Work out the finished part from the listing and answer in its coordinate system (mm). A direction names the side the tool comes from. Round coordinates to 2 decimals unless told otherwise and drop trailing zeros. Write each loop counter-clockwise with the first axis right and the second up, starting at its lowest first coordinate (ties: lowest second). Pieces come first, ordered by that corner, then holes. Notation, with made-up numbers: (-21.5, 9) - (11.5, 9) arc R10 cw to (11.5, 13) - close; hole circle Ø10 at (70, 14.5). An arc over 180 degrees is marked (long way). Write item = value, one per line. Start each with the question number.
from build123d import *

# Parameters (mm, degrees)
EXTRUDE1_DEPTH = 8


with BuildPart() as part:
    # Sketch1 → Extrude1 (new body)
    with BuildSketch(Plane(origin=(0, 0, 0), x_dir=(1, 0, 0), z_dir=(0, 1, 0))):
        Polygon((30, 0), (15, 25.980762114), (-15, 25.980762114), (-30, 0), (-15, -25.980762114), (15, -25.980762114), align=None)
    extrude(amount=EXTRUDE1_DEPTH)

    # Sketch2 → Loft1 section 0
    with BuildSketch(Plane(origin=(0, 8, 0), x_dir=(1, 0, 0), z_dir=(0, 1, 0))):
        Polygon((30, 0), (15, 25.980762114), (-15, 25.980762114), (-30, 0), (-15, -25.980762114), (15, -25.980762114), align=None)
    # Sketch3 → Loft1 section 1
    with BuildSketch(Plane(origin=(0, 43, 0), x_dir=(-1, 0, 0), z_dir=(0, 1, 0))):
        Polygon((20, 0), (10, 17.320508076), (-10, 17.320508076), (-20, 0), (-10, -17.320508076), (10, -17.320508076), align=None)
    loft()

    # Sketch4 → Revolve1 (revolve)
    with BuildSketch(Plane.XY, mode=Mode.PRIVATE) as revolve1_sk:
        Polygon((35, 103), (15, 43), (13.945907447, 43), (33.945907447, 103), align=None)
    revolve(revolve1_sk.sketch.rotate(Axis((0, 43, 0), (0, 1, 0)), 270), axis=Axis((0, 43, 0), (0, 1, 0)))  # turned: the seam where the file's is


solid = part.part
1. Consider line 1 (X direction, y = 60.5, z = -12.5); line 2 (X direction, y = 80, z = -1.5); line 3 (Z direction, x = -13, y = 85). Determine where each line is inside the solid, lowest interval first.
2. Find section A-A on y = 72. Give the vertices of the cut face in (x, z), plus the area to 3 significant figures.
3. Each of these flat-tipped pins is pushed along its axis until it touches: pin 1 (1 mm diameter, centred on y = 63.5, z = -4.5, fed in from +X); pin 2 (6.5 mm diameter, centred on x = -7.5, y = 4.5, fed in from +Z); pin 3 (22.5 mm diameter, centred on x = 1, z = 0, fed in from +Y); pin 4 (10 mm diameter, centred on x = -7, z = -12.5, fed in from -Y). Where does it stop, or does it pass through?
4. For a pull along X with two mould halves and no side action, classify faces 6 (the face through (0, 4, 25.981)), 7 (the face through (22.605, 3.944, -12.809)), 8 (the face through (-22.395, 3.944, -13.172)), 9 (the face through (0, 43, 0)) as released by +X, released by -X, zero draft, split by the parting line, or undercut.
5. Find section B-B on y = 46.5. Give the vertices of the cut face in (x, z).
6. Which of the six approach directions +Z, -Z, +X, -X, +Y, -Y give full straight-line access (tool end or side, diameter ignored) to faces 1 (the face through (22.395, 3.944, 13.172)), 2 (the face through (22.445, 65.913, -2.947)), 3 (the face through (-22.605, 3.944, 12.809)), 4 (the face through (0, 0, 0)), 5 (the face through (0, 4, -25.981))?
Answer key:
q1.line_1 = -16.67 to -15.33, 15.33 to 16.67
q1.line_2 = -27.29 to -26.24, 26.24 to 27.29
q1.line_3 = -25.92 to -24.74, 24.74 to 25.92
q2.outline = circle Ø49.33 at (0, 0); hole circle Ø47.23 at (0, 0)
q2.area = 160 mm²
q3.pin_1 = 21.56
q3.pin_2 = 25.98
q3.pin_3 = 43
q3.pin_4 = 0
q4.face_6 = zero draft
q4.face_7 = released by +X
q4.face_8 = released by -X
q4.face_9 = undercut
q5.outline = circle Ø32.33 at (0, 0); hole circle Ø30.23 at (0, 0)
q6.face_1 = +Z, +X, -Y
q6.face_2 = none
q6.face_3 = +Z, -X, -Y
q6.face_4 = +Z, -Z, +X, -X, -Y
q6.face_5 = -Z, +X, -X, -Y
